Geometry: final body of the model. Coordinates: model frame, mm. A direction names the side the tool comes from. Round coordinates to 2 decimals unless told otherwise and drop trailing zeros. Write each loop counter-clockwise with the first axis right and the second up, starting at its lowest first coordinate (ties: lowest second). Pieces come first, ordered by that corner, then holes. Notation, with made-up numbers: (86, 67) -> (136, 67) arc R32 ccw to (136, 104) -> close; hole circle Ø5 at (78, 6). An arc over 180 degrees is marked (long way). Use one line per item in the form item = value. Start each with the question number.
1. Cut plane A-A, the plane y = 20. Return the cut outline in (x, z), plus the area to 3 significant figures.
2. Cut plane B-B, the plane x = -51.5. Return the cut outline in (y, z).
3. Pin query (flat end, axial travel): pin 1 Ø6 at (x, z) = (-29, -47) entering from -Y; pin 2 Ø4 at (x, z) = (-10, 43) entering from +Y; pin 3 Ø5 at (y, z) = (20.5, -13.5) entering from +X. Return the tip coordinate at first contact, or that it passes through.
4. Draft query along Z for faces 1 (the face through (-30, 33, -55.878)), 2 (the face through (-30, 40, -17.878)), 3 (the face through (-7, 0, 2)). Return one class per face: pulls with the +Z half, pulls with the -Z half, needs draft (parallel to the pull), parting line crosses it, or undercut.
5. Reachability of faces 4 (the face through (-7, 48, 48)), 5 (the face through (-30, 39, -43.878)), 6 (the face through (-30, 0.461, -50)) from +Z, -Z, +X, -X, +Y, -Y: full face, straight path, thin tool, end or side. Return the list, or none.
6. Cut plane D-D, the plane z = 27. Return the cut outline in (x, y).
7. Line query: L1, parallel to X at y = 11, z = 12; L2, parallel to Z at x = -13.5, y = 19.5; L3, parallel to Z at x = -18.5, y = 38.5. Output: solid intervals per line, ascending.
8. Cut plane C-C, the plane x = -30. Return the cut outline in (y, z), plus the area to 3 significant figures.
```python
from build123d import *

# Parameters (mm, degrees)
SKETCH1_R           = 10
BOSS_EXTRUDE1_DEPTH = 14
BOSS_EXTRUDE2_DEPTH = 64
SKETCH4_W           = 60
SKETCH4_H           = 12
BOSS_EXTRUDE4_DEPTH = 64


with BuildPart() as part:
    # Sketch1 → Boss-Extrude1 (new body)
    with BuildSketch(Plane(origin=(0, 0, 0), x_dir=(0, 0, -1), z_dir=(1, 0, 0))):
        with BuildLine():
            ThreePointArc((17.877672838, 50.460908485), (30.877672838, 37.460908485), (43.877672838, 50.460908485))
            Line((43.877672838, 50.460908485), (43.877672838, 64.460908485))
            Line((43.877672838, 64.460908485), (55.877672838, 64.460908485))
            Line((55.877672838, 64.460908485), (55.877672838, 0))
            Line((55.877672838, 0), (-61.381998564, 0))
            Line((-61.381998564, 0), (-61.381998564, 48))
            Line((-61.381998564, 48), (-33.381998564, 48))
            Line((-33.381998564, 48), (-8.122327162, 64.460908485))
            Line((-8.122327162, 64.460908485), (17.877672838, 64.460908485))
            Line((17.877672838, 64.460908485), (17.877672838, 50.460908485))
        make_face()
        with Locations((-46.381998564, 20)):
            Circle(SKETCH1_R, mode=Mode.SUBTRACT)
    extrude(amount=-BOSS_EXTRUDE1_DEPTH)


with BuildPart() as body_2:
    # Mirror4: mirrored copy
    add(part.part.mirror(Plane.ZY.offset(30)))


with BuildPart() as part_1:
    add(part.part)

    add(body_2.part)  # Boss-Extrude2 merges body 2
    # Sketch2 → Boss-Extrude2 (add)
    with BuildSketch(Plane(origin=(0, 64.460908485, 0), x_dir=(1, 0, 0), z_dir=(0, 1, 0))):
        with BuildLine():
            Line((-14, 17.877672838), (-46, 17.877672838))
            Line((-46, 17.877672838), (-60, 17.877672838))
            Line((-60, 17.877672838), (-60, -8.122327162))
            Line((-60, -8.122327162), (-46, -8.122327162))
            ThreePointArc((-46, -8.122327162), (-30, 7.877672838), (-14, -8.122327162))
            Line((-14, -8.122327162), (0, -8.122327162))
            Line((0, -8.122327162), (0, 17.877672838))
            Line((0, 17.877672838), (-14, 17.877672838))
        make_face()
    extrude(amount=-BOSS_EXTRUDE2_DEPTH)

    # Sketch4 → Boss-Extrude4 (add)
    with BuildSketch(Plane(origin=(0, 64.460908485, 0), x_dir=(1, 0, 0), z_dir=(0, 1, 0))):
        with Locations((-30, 49.877672838)):
            Rectangle(SKETCH4_W, SKETCH4_H)
    extrude(amount=-BOSS_EXTRUDE4_DEPTH)


solid = part_1.part
```
Outcome:
q1.outline = (-60, -55.88) -> (0, -55.88) -> (0, 36.38) -> (-14, 36.38) -> (-14, 8.12) arc R16 cw to (-46, 8.12) -> (-46, 36.38) -> (-60, 36.38) -> close; (-60, 56.38) -> (-46, 56.38) -> (-46, 61.38) -> (-60, 61.38) -> close; (-14, 56.38) -> (0, 56.38) -> (0, 61.38) -> (-14, 61.38) -> close; hole (-46, -43.88) -> (-14, -43.88) -> (-14, -17.88) -> (-46, -17.88) -> close
q1.area = 3,540 mm^2
q2.outline = (0, -55.88) -> (64.46, -55.88) -> (64.46, -43.88) -> (50.46, -43.88) arc R13 cw to (50.46, -17.88) -> (64.46, -17.88) -> (64.46, 8.12) -> (48, 33.38) -> (48, 61.38) -> (0, 61.38) -> close; hole circle Ø20 at (20, 46.38)
q3.pin_1 = 0.46
q3.pin_2 = 48
q3.pin_3 = 0
q4.face_1 = pulls with the -Z half
q4.face_2 = undercut
q4.face_3 = needs draft
q5.face_4 = +Z, +X, -X, +Y
q5.face_5 = +Y
q5.face_6 = +Z, -Z, -Y
q6.outline = (-60, 0) -> (-46, 0) -> (-46, 52.16) -> (-60, 52.16) -> close; (-14, 0) -> (0, 0) -> (0, 52.16) -> (-14, 52.16) -> close
q7.L1 = -60 to -46, -14 to 0
q7.L2 = -55.88 to 36.39, 56.37 to 61.38
q7.L3 = -55.88 to -43.88, -17.88 to -3
q8.outline = (0.46, -55.88) -> (64.46, -55.88) -> (64.46, -43.88) -> (0.46, -43.88) -> close; (0.46, -17.88) -> (64.46, -17.88) -> (64.46, -7.88) -> (0.46, -7.88) -> close
q8.area = 1,410 mm^2
